Autodesk Inventor part; units mm, degrees
ref_plane "YZ Plane" through (0, 0, 0) normal (1, 0, 0) x (0, 1, 0)
ref_plane "XZ Plane" through (0, 0, 0) normal (0, 1, 0) x (-1, 0, 0)
ref_plane "XY Plane" through (0, 0, 0) normal (0, 0, 1) x (1, 0, 0)
sketch "Sketch1" plane through (0, 0, 0) normal (1, 0, 0) x (0, 1, 0)
  line L0 (3.2531, 52.0584) -> (0.3531, 52.0584)
  line L1 (0.3531, 52.0584) -> (0.3531, -10.0416)
  line L2 (0.3531, -10.0416) -> (3.2531, -10.0416)
  line L3 (3.2531, -10.0416) -> (3.2531, 52.0584)
  arc A0 (3.2531, 52.0584) -> (2.9699, 57.9259) centre (1.8031, 54.929) ccw
  arc A1 (0.7699, 57.9745) -> (0.3531, 52.0584) centre (1.8031, 54.929) ccw
  line L4 (0.7699, 57.9745) -> (0.7699, 56.8745)
  line L5 (2.9699, 57.9259) -> (2.9699, 56.8259)
  arc A2 (0.7699, 56.8745) -> (2.9699, 56.8259) centre (1.8253, 54.832) ccw
  point P0 (0, 0)
  dimension "d0" = 2.9
  dimension "d1" = 62.1
  dimension "d156" = 1.1
  dimension "d157" = 1.1
  dimension "d158" = 2.2
extrude "Extrusion1" add sketch "Sketch1" against normal blind 20
sketch "Sketch3" plane through (0, 0, 0) normal (1, 0, 0) x (0, 0, -1)
  arc A0 (-52.0584, 3.2531) -> (-57.9259, 2.9699) centre (-54.929, 1.8031) ccw
  line L0 (10.0416, 0.3531) -> (-52.0584, 0.3531)
  line L1 (-52.0584, 3.2531) -> (10.0416, 3.2531)
  line L2 (10.0416, 3.2531) -> (10.0416, 0.3531)
  line L3 (10.0416, 0.3531) -> (-52.0584, 0.3531)
  line L4 (-52.0584, 0.3531) -> (-52.0584, 3.2531)
  point P0 (0, 0)
extrude "Extrusion2" add sketch "Sketch3" along normal blind 42.1
sketch "Sketch4" plane through (42.1, 0, 0) normal (1, 0, 0) x (0, 0, -1)
  line L0 (10.0416, 0.3531) -> (-52.0584, 0.3531)
  line L1 (10.0416, 0.3531) -> (-52.0584, 0.3531)
  line L2 (-52.0584, 0.3531) -> (-52.0584, 3.2531)
  line L3 (-52.0584, 3.2531) -> (10.0416, 3.2531)
  line L4 (10.0416, 3.2531) -> (10.0416, 0.3531)
  arc A0 (-57.9745, 0.7699) -> (-52.0584, 0.3531) centre (-54.929, 1.8031) ccw
  arc A1 (-57.9745, 0.7699) -> (-52.0584, 0.3531) centre (-54.929, 1.8031) ccw
  arc A2 (-52.0584, 3.2531) -> (-57.9259, 2.9699) centre (-54.929, 1.8031) ccw
  arc A3 (-52.0584, 3.2531) -> (-57.9259, 2.9699) centre (-54.929, 1.8031) ccw
  arc A4 (-56.8745, 0.7699) -> (-56.8259, 2.9699) centre (-54.832, 1.8253) ccw
  arc A5 (-56.8745, 0.7699) -> (-56.8259, 2.9699) centre (-54.832, 1.8253) ccw
  line L5 (-56.8745, 0.7699) -> (-57.9745, 0.7699)
  line L6 (-56.8745, 0.7699) -> (-57.9745, 0.7699)
  line L7 (-57.9259, 2.9699) -> (-56.8259, 2.9699)
  line L8 (-56.8259, 2.9699) -> (-57.9259, 2.9699)
  point P0 (0, 0)
  dimension "d159" = 1.1
  dimension "d160" = 2.2
extrude "Extrusion3" add sketch "Sketch4" along normal blind 20
sketch "Sketch9" plane through (0, 0.3531, 52.0584) normal (0, 0, 1) x (1, 0, 0)
  line L0 (0, 2.9) -> (42.1, 2.9)
  line L1 (0, 2.9) -> (42.1, 2.9)
  line L2 (42.1, 2.9) -> (42.1, 0)
  line L3 (42.1, 0) -> (0, 0)
  line L4 (0, 0) -> (0, 2.9)
  point P0 (0, -0.3531)
extrude "Extrusion4" add sketch "Sketch9" along normal blind 6
sketch "Sketch10" plane through (-20, 0, 0) normal (-1, 0, 0) x (0, 0, 1)
  arc A0 (52.0584, 0.3531) -> (57.9745, 0.7699) centre (54.929, 1.8031) ccw
  line L0 (-10.0416, 3.2531) -> (-10.0416, 0.3531)
  line L1 (52.0584, 0.3531) -> (-10.0416, 0.3531)
  line L2 (-10.0416, 0.3531) -> (-10.0416, 3.2531)
  line L3 (-10.0416, 3.2531) -> (52.0584, 3.2531)
  line L4 (52.0584, 3.2531) -> (52.0584, 0.3531)
  point P0 (0, 0)
extrude "Extrusion5" add sketch "Sketch10" along normal blind 8.95
sketch "Sketch11" plane through (62.1, 0, 0) normal (1, 0, 0) x (0, 0, -1)
  line L0 (10.0416, 0.3531) -> (10.0416, 3.2531)
  arc A0 (-52.0584, 3.2531) -> (-57.7996, 3.2531) centre (-54.929, 1.8031) ccw
  line L1 (10.0416, 0.3531) -> (-52.0584, 0.3531)
  line L2 (-52.0584, 0.3531) -> (-52.0584, 3.2531)
  line L3 (-52.0584, 3.2531) -> (10.0416, 3.2531)
  line L4 (10.0416, 3.2531) -> (10.0416, 0.3531)
  point P0 (0, 0)
extrude "Extrusion6" add sketch "Sketch11" along normal blind 8.95
sketch "Sketch5" plane through (-20, 0.3531, -10.0416) normal (0, -1, 0) x (1, 0, 0)
  line L0 (20, 62.1) -> (62.1, 62.1)
  line L1 (0, 0) -> (0, 62.1)
  line L2 (62.1, 68.1) -> (20, 68.1)
  line L3 (-8.95, 0) -> (-8.95, 62.1)
  point P0 (20, 10.0416)
  point P1 (29.15, 60.6)
  dimension "d80" = 38.1
  dimension "d81" = 7.5
hole "Hole1" at (9.15, 0.3531, 50.5584) direction (0, 1, 0) diameter 2.921 end through all
sketch "Sketch6" plane through (-20, 0.3531, -10.0416) normal (0, -1, 0) x (1, 0, 0)
  line L0 (20, 62.1) -> (62.1, 62.1)
  circle A0 centre (29.15, 60.6) radius 1.4605
  line L1 (62.1, 68.1) -> (20, 68.1)
  point P0 (20, 10.0416)
  point P1 (52.95, 60.6)
  dimension "d42" = 23.8
  dimension "d53" = 7.5
hole "Hole2" at (32.95, 0.3531, 50.5584) direction (0, 1, 0) diameter 2.921 end through all
sketch "Sketch7" plane through (-20, 0.3531, -10.0416) normal (0, -1, 0) x (1, 0, 0)
  line L0 (0, 0) -> (0, 62.1)
  circle A0 centre (29.15, 60.6) radius 1.4605
  line L1 (-8.95, 0) -> (-8.95, 62.1)
  point P0 (20, 10.0416)
  point P1 (29.15, 2.71)
  dimension "d49" = 57.89
  dimension "d82" = 38.1
hole "Hole3" at (9.15, 0.3531, -7.3316) direction (0, 1, 0) diameter 2.921 end through all
sketch "Sketch8" plane through (-20, 0.3531, -10.0416) normal (0, -1, 0) x (1, 0, 0)
  circle A0 centre (29.15, 2.71) radius 1.4605
  circle A1 centre (52.95, 60.6) radius 1.4605
  point P0 (20, 10.0416)
  point P1 (52.95, 2.71)
  point P2 (41.1972, 0)
  point P3 (38.7028, 0)
  point P4 (60, 64.989)
  point P5 (60, 63.311)
  dimension "d48" = 23.8
  dimension "d54" = 57.89
hole "Hole4" at (32.95, 0.3531, -7.3316) direction (0, 1, 0) diameter 2.921 end through all
sketch "Sketch12" plane through (0, 0.3531, 58.0584) normal (0, -1, 0) x (1, 0, 0)
  line L0 (-20, -6) -> (-28.95, -6)
  line L1 (-28.95, -68.1) -> (-28.95, -6)
  point P0 (0, -58.0584)
  point P1 (-23.54, -14.57)
  dimension "d133" = 8.57
  dimension "d134" = 5.41
hole "Hole5" at (-23.54, 0.3531, 43.4884) direction (0, 1, 0) diameter 2.921 end through all
sketch "Sketch13" plane through (0, 0.3531, 58.0584) normal (0, -1, 0) x (1, 0, 0)
  line L0 (0, -6) -> (-20, -6)
  circle A0 centre (-23.54, -14.57) radius 1.4605
  point P0 (0, -58.0584)
  point P1 (-10.28, -14.57)
  dimension "d135" = 8.57
  dimension "d136" = 13.26
hole "Hole6" at (-10.28, 0.3531, 43.4884) direction (0, 1, 0) diameter 2.921 end through all
sketch "Sketch14" plane through (0, 0.3531, 58.0584) normal (0, -1, 0) x (1, 0, 0)
  line L0 (-28.95, -68.1) -> (-28.95, -6)
  circle A0 centre (-23.54, -14.57) radius 1.4605
  point P0 (0, -58.0584)
  point P1 (-23.54, -59.53)
  dimension "d137" = 5.41
  dimension "d138" = 44.96
hole "Hole7" at (-23.54, 0.3531, -1.4716) direction (0, 1, 0) diameter 2.921 end through all
sketch "Sketch15" plane through (0, 0.3531, 58.0584) normal (0, -1, 0) x (1, 0, 0)
  circle A0 centre (-10.28, -14.57) radius 1.4605
  circle A1 centre (-23.54, -59.53) radius 1.4605
  point P0 (0, -58.0584)
  point P1 (-10.28, -59.53)
  dimension "d139" = 44.96
  dimension "d148" = 13.26
hole "Hole8" at (-10.28, 0.3531, -1.4716) direction (0, 1, 0) diameter 2.921 end through all
sketch "Sketch17" plane through (0, 0.3531, 58.0584) normal (0, -1, 0) x (1, 0, 0)
  line L0 (71.05, -6) -> (71.05, -68.1)
  line L1 (62.1, -6) -> (71.05, -6)
  point P0 (0, -58.0584)
  point P1 (65.64, -14.57)
  dimension "d142" = 5.41
  dimension "d147" = 8.57
hole "Hole10" at (65.64, 0.3531, 43.4884) direction (0, 1, 0) diameter 2.921 end through all
sketch "Sketch16" plane through (0, 0.3531, 58.0584) normal (0, -1, 0) x (1, 0, 0)
  circle A0 centre (65.64, -14.57) radius 1.4605
  line L0 (42.1, -6) -> (62.1, -6)
  point P0 (0, -58.0584)
  point P1 (52.38, -14.57)
  dimension "d144" = 13.26
  dimension "d146" = 8.57
hole "Hole9" at (52.38, 0.3531, 43.4884) direction (0, 1, 0) diameter 2.921 end through all
sketch "Sketch19" plane through (0, 0.3531, 58.0584) normal (0, -1, 0) x (1, 0, 0)
  circle A0 centre (65.64, -14.57) radius 1.4605
  line L0 (71.05, -6) -> (71.05, -68.1)
  point P0 (0, -58.0584)
  point P1 (65.64, -59.53)
  dimension "d141" = 44.96
  dimension "d143" = 5.41
hole "Hole12" at (65.64, 0.3531, -1.4716) direction (0, 1, 0) diameter 2.921 end through all
sketch "Sketch18" plane through (0, 0.3531, 58.0584) normal (0, -1, 0) x (1, 0, 0)
  circle A0 centre (52.38, -14.57) radius 1.4605
  circle A1 centre (65.64, -59.53) radius 1.4605
  point P0 (0, -58.0584)
  point P1 (52.38, -59.53)
  dimension "d140" = 44.96
  dimension "d145" = 13.26
hole "Hole11" at (52.38, 0.3531, -1.4716) direction (0, 1, 0) diameter 2.921 end through all
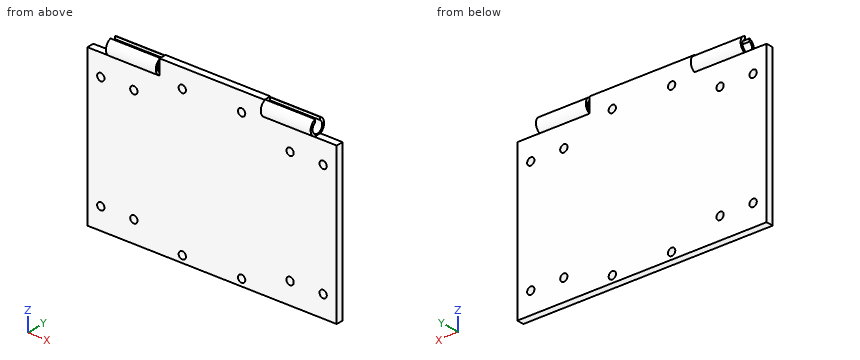
Design review of the part built by this model. Coordinates are the model's own, in mm. Give positions to 0.01 mm unless a question says otherwise; leave off trailing zeros. Write each loop counter-clockwise with the first axis right and the second up, starting at its lowest first coordinate (ties: lowest second). Pieces come first, ordered by that corner, then holes. Notation, with made-up numbers: (5.25, 88) - (28.25, 88) arc R18 cw to (28.25, 121) - close; hole circle Ø3 at (30, -26). An arc over 180 degrees is marked (long way). Return JSON: item names as keys, results as strings. Group by question number.
(1) We need section D-D, the plane x = 36.5. Give the boundary of the cut face in (y, z), then the cut area to 3 significant figures.
(2) We need section C-C, the plane z = 36.5. Give the boundary of the cut face in (x, y), then the cut area to 3 significant figures.
(3) Insertion check: pin 1 (3.5 mm diameter, centred on x = -10.28, z = 43.49, fed in from -Y); pin 2 (1.5 mm diameter, centred on y = 1.5, z = 54, fed in from -X); pin 3 (0.9 mm diameter, centred on x = -7, z = 57.5, fed in from -Y). Each pin has a flat end and moves straight along its axis. Give the tip position at first contact, or say it passes through.
(4) To check wall thickness, follow probe 1 along Z at (x, y) = (65.64, 1.1); probe 2 along Z at (x, y) = (-10.28, 1.65); probe 3 along X at (y, z) = (0.75, -6). State the ranges of each line that lie inside material, in increasing order.
(5) We need section B-B, the plane x = 9.15. Give the boundary of the cut face in (y, z), then the cut area to 3 significant figures.
(6) We need section A-A, the plane x = 65.64. Give the boundary of the cut face in (y, z), then the cut area to 3 significant figures.
Reported:
{
 "1": {"outline": "(0.35, -10.04) - (3.25, -10.04) - (3.25, 58.06) - (0.35, 58.06) - close", "area": "197 mm2"},
 "2": {"outline": "(-28.95, 0.35) - (71.05, 0.35) - (71.05, 3.25) - (-28.95, 3.25) - close", "area": "290 mm2"},
 "3": {"pin 1": "stops at y = 0.35", "pin 2": "stops at x = 0", "pin 3": "stops at y = -0.61"},
 "4": {"probe 1": "z = -10.04 to -2.93, -0.01 to 42.03, 44.95 to 52.06", "probe 2": "z = -10.04 to -2.93, -0.01 to 42.03, 44.95 to 52.54", "probe 3": "x = -28.95 to 8.55, 9.75 to 32.35, 33.55 to 71.05"},
 "5": {"outline": "(0.35, -10.04) - (3.25, -10.04) - (3.25, -8.79) - (0.35, -8.79) - close; (0.35, -5.87) - (3.25, -5.87) - (3.25, 49.1) - (0.35, 49.1) - close; (0.35, 52.02) - (3.25, 52.02) - (3.25, 58.06) - (0.35, 58.06) - close", "area": "181 mm2"},
 "6": {"outline": "(0.35, -10.04) - (3.25, -10.04) - (3.25, -2.93) - (0.35, -2.93) - close; (0.35, -0.01) - (3.25, -0.01) - (3.25, 42.03) - (0.35, 42.03) - close; (0.35, 44.95) - (3.25, 44.95) - (3.25, 52.06) - (0.35, 52.06) - close", "area": "163 mm2"}
}
